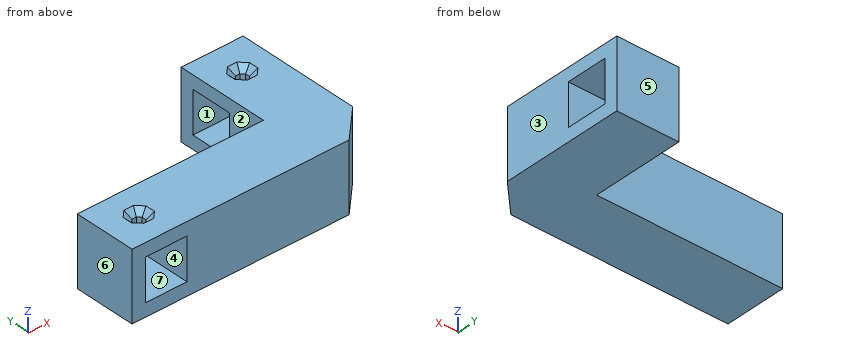
from build123d import *

# Parameters (mm, degrees)
PAD_DEPTH       = 22
SKETCH001_W     = 13.45
SKETCH001_H     = 13.45
POCKET_DEPTH    = 20.001
SKETCH002_W     = 13.45
SKETCH002_H     = 13.45
POCKET001_DEPTH = 15
CHAMFER_SIZE    = 10
POCKET002_DEPTH = 5
CHAMFER001_SIZE = 2


with BuildPart() as part:
    # Sketch → Pad (new body)
    with BuildSketch(Plane.XY):
        Polygon((0, 30), (0, 0), (-60, 0), (-60, -20), (20, -20), (20, 30), align=None)
    extrude(amount=PAD_DEPTH)

    # Sketch001 (on Face1 of Pad) → Pocket (cut, through all)
    with BuildSketch(Plane(origin=(0, 0, 0), x_dir=(0, -1, 0), z_dir=(-1, 0, 0))):
        with Locations((-19, 11)):
            Rectangle(SKETCH001_W, SKETCH001_H)
    extrude(amount=-POCKET_DEPTH, mode=Mode.SUBTRACT)

    # Sketch002 (on Face12 of Pocket) → Pocket001 (cut)
    with BuildSketch(Plane.XZ.offset(20)):
        with Locations((-49, 11)):
            Rectangle(SKETCH002_W, SKETCH002_H)
    extrude(amount=-POCKET001_DEPTH, mode=Mode.SUBTRACT)

    # Chamfer
    chamfer_edges = [part.edges().sort_by_distance(p)[0] for p in [
        (20, -20, 11),
    ]]
    chamfer(chamfer_edges, length=CHAMFER_SIZE)

    # Sketch003 (on Face9 of Chamfer) → Pocket002 (cut)
    with BuildSketch(Plane.XY.offset(22)):
        Polygon((9.295837, 17.3), (10.704163, 17.3), (11.7, 18.295837), (11.7, 19.704163), (10.704163, 20.7), (9.295837, 20.7), (8.3, 19.704163), (8.3, 18.295837), align=None)
        Polygon((-47.3, -10.704163), (-47.3, -9.295837), (-48.295837, -8.3), (-49.704163, -8.3), (-50.7, -9.295837), (-50.7, -10.704163), (-49.704163, -11.7), (-48.295837, -11.7), align=None)
    extrude(amount=-POCKET002_DEPTH, mode=Mode.SUBTRACT)

    # Chamfer001
    chamfer001_edges = [part.edges().sort_by_distance(p)[0] for p in [
        (-50.7, -10, 22),
        (-50.202082, -8.797918, 22),
        (-49, -8.3, 22),
        (-47.797918, -8.797918, 22),
        (-47.3, -10, 22),
        (-47.797918, -11.202082, 22),
        (-49, -11.7, 22),
        (-50.202082, -11.202082, 22),
        (8.3, 19, 22),
        (8.797918, 20.202082, 22),
        (10, 20.7, 22),
        (11.202082, 20.202082, 22),
        (11.7, 19, 22),
        (11.202082, 17.797918, 22),
        (10, 17.3, 22),
        (8.797918, 17.797918, 22),
    ]]
    chamfer(chamfer001_edges, length=CHAMFER001_SIZE)


solid = part.part
Read the model definition and answer for the solid it produces. Units are mm, in the model's axes. Face numbers are marked on the shaded views. A direction names the side the tool comes from. Round coordinates to 2 decimals unless told otherwise and drop trailing zeros. Loops run counter-clockwise (first coordinate to the right, second up) from the corner with the lowest first, then second, coordinate; pieces in that order, holes last.
Q1. Each of these flat-tipped pins is pushed along its axis until it touches: pin 1 (1.5 mm diameter, centred on y = 19, z = 19.5, fed in from -X); pin 2 (11 mm diameter, centred on x = -50, y = -16, fed in from -Z); pin 3 (1 mm diameter, centred on y = 13, z = 16.5, fed in from -X); pin 4 (11 mm diameter, centred on x = -33.5, z = 11, fed in from +Y). Where does it stop, or does it pass through?
Q2. Determine the mould class of the marked faces 4, 5, 6 and 7 for opening direction X: released by +X, released by -X, zero draft, split by the parting line, or undercut.
Q3. Which of the six approach directions +Z, -Z, +X, -X, +Y, -Y give full straight-line access (tool end or side, diameter ignored) to the marked faces 1, 2 and 3?
Q4. Section D-D on y = 3.5 is taken. Write down the section's boundary in (x, z), and give its area (3 significant figures).
Q5. Section B-B on z = 5.5 is taken. Write down the section's boundary in (x, y) (3 decimals).
Q6. Section C-C on x = -19 is taken. Write down the section's boundary in (y, z).
Q7. Section A-A on y = 14 is taken. Write down the section's boundary in (x, z) (3 decimals), and give its area (3 significant figures).
Q8. Consider probe 1 along Z at (x, y) = (3.5, 14.5) (3 decimals); probe 2 along X at (y, z) = (-9.5, 18.25); probe 3 along X at (y, z) = (8.5, 11.5). Determine where each line is inside the solid, lowest interval first.
Output:
1. pin 1: stops at x = 0
1. pin 2: stops at z = 0
1. pin 3: passes through
1. pin 4: stops at y = 0
2. face 4: undercut
2. face 5: zero draft
2. face 6: released by -X
2. face 7: undercut
3. face 1: +X, -X
3. face 2: +Z, -Z, -X, +Y
3. face 3: +Z, -Z, +X, +Y, -Y
4. outline: (0, 0) - (20, 0) - (20, 22) - (0, 22) - close
4. area: 440 mm2
5. outline: (-60, -20) - (-55.725, -20) - (-55.725, -5) - (-42.275, -5) - (-42.275, -20) - (10, -20) - (20, -10) - (20, 12.275) - (0, 12.275) - (0, 0) - (-60, 0) - close; (0, 25.725) - (20, 25.725) - (20, 30) - (0, 30) - close
6. outline: (-20, 0) - (0, 0) - (0, 22) - (-20, 22) - close
7. outline: (0, 0) - (20, 0) - (20, 4.275) - (0, 4.275) - close; (0, 17.725) - (20, 17.725) - (20, 22) - (0, 22) - close
7. area: 171 mm2
8. probe 1: z = 0 to 4.275, 17.725 to 22
8. probe 2: x = -60 to -50.7, -47.3 to 20
8. probe 3: x = 0 to 20
